The model under review builds one solid part; all positions refer to its coordinate system, in mm. A direction names the side the tool comes from. Coordinates: 2 decimals unless noted, no trailing zeros. Loops run counter-clockwise (first coordinate to the right, second up) from the corner with the lowest first, then second, coordinate; pieces in that order, holes last. Notation, with made-up numbers: (33.25, -19.5) - (69.25, -19.5) arc R24 cw to (69.25, -4.5) - close; hole circle Ø4 at (69, 15.25). An arc over 180 degrees is marked (long way). Answer in a Markdown table with one row per item. Add a question column.
(1) For line 1 along Y through (x, z) = (-23.5, 18); line 2 along Z through (x, y) = (-10, 49.5), list the stretches that pass through material, from the lowest coordinate up.
(2) For P1, Ø4, axis at y = 54, z = 49, coming from the -X side; P2, Ø4, axis at x = -4.5, y = 18, coming from the +Z side; P3, Ø14, axis at y = 14, z = 30, coming from the -X side, all flat-tipped, find the tip position at first contact; note any pin that passes through.
(3) We need section A-A on x = -16. Write out the cut boundary in (y, z).
(4) We need section D-D on x = -56.5. Write out the cut boundary in (y, z).
(5) Machinability: for faces 1 (the flat face through (-36, 21, 44.368)), 2 (the flat face through (-60, 6, 16.752)), 3 (the flat face through (-51, 12, 25)), which of the approach directions +Z, -Z, +X, -X, +Y, -Y give a long, thin tool a straight path to every point of the face, cutting with its end or side? Answer none if there is none.
(6) We need section C-C on z = 7.5. Write out the cut boundary in (x, y), plus the area to 3 significant figures.
(7) We need section B-B on y = 25.5. Write out the cut boundary in (x, z), plus the area to 3 significant figures.
(8) Mouldability with a two-part tool opening along Z and no side actions: class faces 4 (the flat face through (-20, 21, 16.368)), 5 (the flat face through (-70, 48, 8)), 6 (the flat face through (-41, 32, 16)), 7 (the flat face through (-4, 21, 44.368)) as +Z half, -Z half, draft (parallel to the pull), parting line (faces both ways), or undercut.
from build123d import *

# Parameters (mm, degrees)
F0_W      = 80
F0_H      = 64
F1_DEPTH  = 16
F2_W      = 64
F2_H      = 64
F3_DEPTH  = 16
F4_R      = 32
F5_W      = 40
F5_H      = 28
F6_DEPTH  = 42
F8_DEPTH  = 42
F10_DEPTH = 12
F11_W     = 20
F11_H     = 16
F12_DEPTH = 16


with BuildPart() as f1:
    # F0 (on Top) → F1 (new body)
    with BuildSketch(Plane.XY):
        with Locations((-40, 32)):
            Rectangle(F0_W, F0_H)
    extrude(amount=F1_DEPTH)

    # F2 (on Right) → F3 (join)
    with BuildSketch(Plane.YZ):
        with Locations((32, 32)):
            Rectangle(F2_W, F2_H)
    extrude(amount=F3_DEPTH)

    # F4
    f4_edges = [f1.edges().sort_by_distance(p)[0] for p in [
        (8, 64, 64),
    ]]
    fillet(f4_edges, radius=F4_R)

    # F5 (on Front) → F6 (join)
    with BuildSketch(Plane.XZ):
        with Locations((-20, 30.368277)):
            Rectangle(F5_W, F5_H)
    extrude(amount=-F6_DEPTH)

    # F7 (on face) → F8 (cut)
    with BuildSketch(Plane(origin=(0, 42, 0), x_dir=(-1, 0, 0), z_dir=(0, 1, 0))):
        with BuildLine():
            Line((32, 44.368277), (8.002928, 44.368277))
            ThreePointArc((8.002928, 44.368277), (20.001464, 32.180844), (32, 44.368277))
        make_face()
    extrude(amount=-F8_DEPTH, mode=Mode.SUBTRACT)

    # F9 (on Front) → F10 (join)
    with BuildSketch(Plane.XZ):
        Polygon((-40, 16.752034), (-40, 44.752034), (-80, 16.752034), align=None)
    extrude(amount=-F10_DEPTH)

    # F11 (on face) → F12 (cut)
    with BuildSketch(Plane.XY.offset(16)):
        with Locations((-70, 40)):
            Rectangle(F11_W, F11_H)
        with BuildLine():
            Line((-60, 48), (-60, 32))
            ThreePointArc((-60, 32), (-52, 40), (-60, 48))
        make_face()
    extrude(amount=-F12_DEPTH, mode=Mode.SUBTRACT)


solid = f1.part
Outcome:
| question | item | result |
|---|---|---|
| 1 | line 1 | 0 to 42 |
| 1 | line 2 | 0 to 16 |
| 2 | P1 | x = 0 |
| 2 | P2 | z = 44.37 |
| 2 | P3 | x = -70.66 |
| 3 | outline | (0, 0) - (64, 0) - (64, 16) - (0, 16) - close; (0, 16.37) - (42, 16.37) - (42, 32.87) - (0, 32.87) - close |
| 4 | outline | (0, 0) - (32.81, 0) - (32.81, 16) - (0, 16) - close; (0, 16.75) - (12, 16.75) - (12, 33.2) - (0, 33.2) - close; (47.19, 0) - (64, 0) - (64, 16) - (47.19, 16) - close |
| 5 | face 1 | +Z, +Y, -Y |
| 5 | face 2 | -X, +Y, -Y |
| 5 | face 3 | +Z, -X, +Y |
| 6 | outline | (-80, 0) - (16, 0) - (16, 64) - (-80, 64) - (-80, 48) - (-60, 48) arc R8 cw to (-60, 32) - (-80, 32) - close |
| 6 | area | 5,720 mm² |
| 7 | outline | (-80, 0) - (16, 0) - (16, 64) - (0, 64) - (0, 44.37) - (-8, 44.37) arc R12 cw (long way) to (-32, 44.37) - (-40, 44.37) - (-40, 16.37) - (0, 16.37) - (0, 16) - (-80, 16) - close |
| 7 | area | 3,190 mm² |
| 8 | face 4 | undercut |
| 8 | face 5 | draft |
| 8 | face 6 | undercut |
| 8 | face 7 | +Z half |
